```python
from build123d import *

# Parameters (mm, degrees)
SKETCH5_W               = 6.477
SKETCH5_H               = 101.6
SKETCH5_W_2             = 101.6
SKETCH5_H_2             = 6.477
BOSS_EXTRUDE1_DEPTH     = 19.05
CUT_EXTRUDE2_DEPTH      = 251.206
CUT_EXTRUDE2_DEPTH_BACK = 164.846


with BuildPart() as part:
    # Sketch2 → Loft1 section 0
    with BuildSketch(Plane(origin=(0, 127, 0), x_dir=(1, 0, 0), z_dir=(0, 1, 0))):
        with BuildLine():
            Line((-50.8, -50.8), (278.13, -50.8))
            Line((278.13, -50.8), (278.13, 276.352))
            Line((278.13, 276.352), (-50.8, 276.352))
            Line((-50.8, 276.352), (-50.8, -50.8))
        make_face()
    # Sketch1 → Loft1 section 1
    with BuildSketch(Plane(origin=(0, 0, 0), x_dir=(1, 0, 0), z_dir=(0, 1, 0))):
        with BuildLine():
            Line((0, 0), (227.33, 0))
            Line((227.33, 0), (227.33, 225.552))
            Line((227.33, 225.552), (0, 225.552))
            Line((0, 225.552), (0, 0))
        make_face()
    loft()

    # Sketch4 → Cut-Loft3 section 0
    with BuildSketch(Plane.XZ):
        with BuildLine():
            Line((208.28, -19.05), (19.05, -19.05))
            Line((19.05, -19.05), (19.05, -206.502))
            Line((19.05, -206.502), (208.28, -206.502))
            Line((208.28, -206.502), (208.28, -19.05))
        make_face()
    # Sketch3 → Cut-Loft3 section 1
    with BuildSketch(Plane(origin=(0, 127, 0), x_dir=(1, 0, 0), z_dir=(0, 1, 0))):
        with BuildLine():
            Line((-31.75, 257.302), (-31.75, -31.75))
            Line((-31.75, -31.75), (259.08, -31.75))
            Line((259.08, -31.75), (259.08, 257.302))
            Line((259.08, 257.302), (-31.75, 257.302))
        make_face()
    loft(mode=Mode.SUBTRACT)

    # Sketch5 → Boss-Extrude1 (add)
    with BuildSketch(Plane.XZ):
        with Locations((3.2385, -112.776)):
            Rectangle(SKETCH5_W, SKETCH5_H)
        with Locations((15.8115, -112.776)):
            Rectangle(SKETCH5_W, SKETCH5_H)
        with Locations((113.665, -2.3495)):
            Rectangle(SKETCH5_W_2, SKETCH5_H_2)
        with Locations((113.665, -14.9225)):
            Rectangle(SKETCH5_W_2, SKETCH5_H_2)
        with Locations((224.0915, -112.776)):
            Rectangle(SKETCH5_W, SKETCH5_H)
        with Locations((211.5185, -112.776)):
            Rectangle(SKETCH5_W, SKETCH5_H)
        with Locations((113.665, -223.2025)):
            Rectangle(SKETCH5_W_2, SKETCH5_H_2)
        with Locations((113.665, -210.6295)):
            Rectangle(SKETCH5_W_2, SKETCH5_H_2)
    extrude(amount=BOSS_EXTRUDE1_DEPTH)

    # Sketch6 → Cut-Extrude2 (cut, two sides: drawn at the far end of the back side and taken through both)
    with BuildSketch(Plane(origin=(0, 0, 0), x_dir=(1, 0, 0), z_dir=(0, 1, 0)).offset(-CUT_EXTRUDE2_DEPTH_BACK)):
        Polygon((278.13, 276.352), (112.012514998, 276.352), (112.838757499, 112.776), (278.13, 112.776), align=None)
        Polygon((278.13, 112.776), (112.838757499, 112.776), (113.665, -50.8), (278.13, -50.8), align=None)
        Polygon((113.665, -50.8), (112.838757499, 112.776), (-50.8, 112.776), (-50.8, -50.8), align=None)
    extrude(amount=CUT_EXTRUDE2_DEPTH + CUT_EXTRUDE2_DEPTH_BACK, mode=Mode.SUBTRACT)


solid = part.part
```
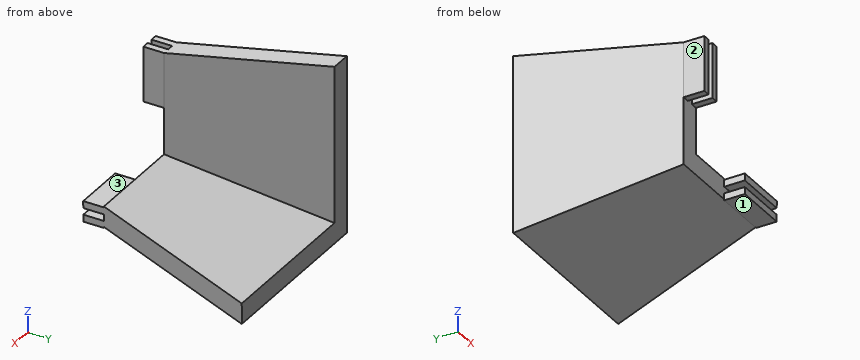
Geometry: final body of the model. Coordinates: model frame, mm. Face numbers are marked on the shaded views. A direction names the side the tool comes from. Round coordinates to 2 decimals unless told otherwise and drop trailing zeros. Use one line per item in the form item = value.
(1) Access query for the marked faces 1, 2 and 3. Directions: +Z, -Z, +X, -X, +Y, -Y. A direction counts if a zero-diameter tool reaches every point of the face in a straight line with its end or side. Return the directions, or none.
Results list:
face_1 = -Z, +X, -X, -Y
face_2 = +Z, -Z, -X, -Y
face_3 = +Z, +X, -X, -Y
(2) First-contact query: pin 1 Ø4 at (y, z) = (89, -253) entering from +X; pin 2 Ø3 at (x, z) = (20.5, -185) entering from +Y (3 decimals); pin 3 Ø1 at (y, z) = (77.5, -181) entering from -X. Flat tips, straight axial feed; report the tip coordinate or a pass-through.
Results list:
pin_1 = 112.14
pin_2 = 0.125
pin_3 = -31.2
(3) Ray query, probe 1 along X at (y, z) = (118.5, -156.5); probe 2 along X at (y, z) = (109.5, -189.5); probe 3 along Z at (x, y) = (105, 87). Return the intervals inside material, ascending. Write a range as [from, to].
Results list:
probe_1 = [-47.4, -28.35]
probe_2 = [-43.8, -24.75]
probe_3 = [-260.35, -241.3]
